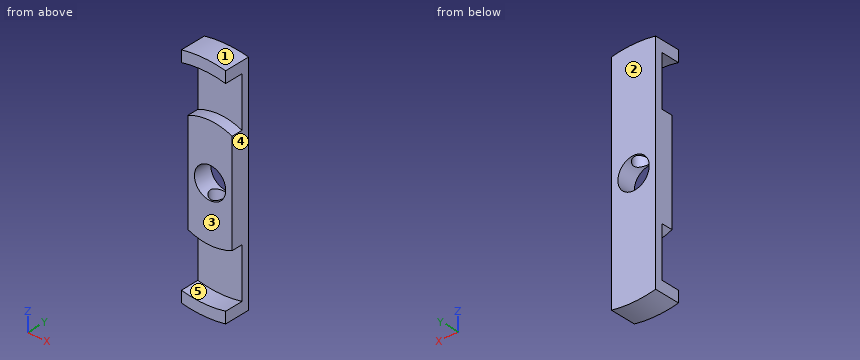
```python
from build123d import *

# Parameters (mm, degrees)
CORTE_EXTRUS_O1_DEPTH      = 45.395945761
CORTE_EXTRUS_O1_DEPTH_BACK = 45.395945761
ESBO_O2_W                  = 96.741183006
ESBO_O2_H                  = 102.357875962
ESBO_O2_W_2                = 12
ESBO_O2_H_2                = 76.270119436
ESBO_O3_R                  = 2.1
CORTE_EXTRUS_O4_DEPTH      = 13


with BuildPart() as part:
    # Esboço1 → Revolução1 (revolve)
    with BuildSketch(Plane.XY, mode=Mode.PRIVATE) as revolu_o1_sk:
        Polygon((4.25, 5), (4.25, 0), (15, 0), (15, 3), (28, 3), (28, -2), (31, -2), (31, 5), align=None)
    revolve(revolu_o1_sk.sketch.rotate(Axis((0, 0, 0), (0, 1, 0)), 90), axis=Axis((0, 0, 0), (0, 1, 0)))

    # Esboço2 → Corte-extrusão1 (cut, two sides: drawn at the far end of the back side and taken through both)
    with BuildSketch(Plane(origin=(0, 5, 0), x_dir=(1, 0, 0), z_dir=(0, 1, 0)).offset(-CORTE_EXTRUS_O1_DEPTH_BACK)):
        Rectangle(ESBO_O2_W, ESBO_O2_H)
        Rectangle(ESBO_O2_W_2, ESBO_O2_H_2, mode=Mode.SUBTRACT)
    extrude(amount=CORTE_EXTRUS_O1_DEPTH + CORTE_EXTRUS_O1_DEPTH_BACK, mode=Mode.SUBTRACT)

    # Esboço3 → Corte-extrusão4 (cut, symmetric)
    with BuildSketch(Plane.XY):
        with Locations((0, 2.5)):
            Circle(ESBO_O3_R)
    extrude(amount=CORTE_EXTRUS_O4_DEPTH, both=True, mode=Mode.SUBTRACT)


solid = part.part
```
The model under review builds one solid part; all positions refer to its coordinate system, in mm. Face numbers are marked on the shaded views. A direction names the side the tool comes from. Round coordinates to 2 decimals unless told otherwise and drop trailing zeros. Loops run counter-clockwise (first coordinate to the right, second up) from the corner with the lowest first, then second, coordinate; pieces in that order, holes last.
1) Wall thickness on line 1 along X through (y, z) = (2.5, -10.5); line 2 along Z through (x, y) = (-2.75, 0.25); line 3 along Z through (x, y) = (5, 2.5): over which ranges is each line inside the solid? List them lowest first.
Values follow:
line 1: x = -6 to -2.1, 2.1 to 6
line 2: z = -30.88 to -27.86, -14.75 to -3.24, 3.24 to 14.75, 27.86 to 30.88
line 3: z = -30.59 to -27.55, -14.14 to 14.14, 27.55 to 30.59
2) The part is to be moulded in two halves that separate along Z. For the marked faces 1, 2 and 3, say which applies: pulls with the +Z half, pulls with the -Z half, needs draft (parallel to the pull), parting line crosses it, or undercut.
Values follow:
face 1: pulls with the +Z half
face 2: needs draft
face 3: undercut
3) Consider section B-B on x = 0. State the section outline as (y, z) points.
Values follow:
outline: (-2, -31) - (5, -31) - (5, -4.25) - (4.6, -4.25) - (4.6, -13) - (0.4, -13) - (0.4, -4.25) - (0, -4.25) - (0, -15) - (3, -15) - (3, -28) - (-2, -28) - close; (-2, 28) - (3, 28) - (3, 15) - (0, 15) - (0, 4.25) - (0.4, 4.25) - (0.4, 13) - (4.6, 13) - (4.6, 4.25) - (5, 4.25) - (5, 31) - (-2, 31) - close
4) Tool access review of the marked faces 4 and 5: name each direction out of +Z, -Z, +X, -X, +Y, -Y from which nothing blocks a thin tool from reaching the whole face with its end or side.
Values follow:
face 4: +Z, -Z, +X, +Y, -Y
face 5: -Y
5) Consider section A-A on z = 0. State the section outline as (x, y) points.
Values follow:
outline: (-6, 0) - (-4.25, 0) - (-4.25, 5) - (-6, 5) - close; (4.25, 0) - (6, 0) - (6, 5) - (4.25, 5) - close
6) Consider section D-D on x = 3.25. State the section outline as (y, z) points, then the cut area to 3 significant figures.
Values follow:
outline: (-2, -30.83) - (5, -30.83) - (5, -2.74) - (0, -2.74) - (0, -14.64) - (3, -14.64) - (3, -27.81) - (-2, -27.81) - close; (-2, 27.81) - (3, 27.81) - (3, 14.64) - (0, 14.64) - (0, 2.74) - (5, 2.74) - (5, 30.83) - (-2, 30.83) - close
area: 214 mm2
7) Consider section C-C on z = -9. State the section outline as (x, y) points.
Values follow:
outline: (-6, 0) - (6, 0) - (6, 5) - (-6, 5) - close; hole circle Ø4.2 at (0, 2.5)
8) Clearance check with flat-ended pins moving along their axes: P1, Ø4, axis at x = -2.5, y = -1, coming from the -Z side; P2, Ø4, axis at x = 0, y = 2.5, coming from the +Z side; P3, Ø1.5, axis at x = 4, y = 1.5, coming from the +Z side. State where each tip first meets the part, or that it passes through.
Values follow:
P1: stops at z = -31
P2: stops at z = 31
P3: stops at z = 30.83
